from build123d import *

# Parameters (mm, degrees)
SZKIC1_W                    = 125
SZKIC1_H                    = 80
DODANIE_WYCI_GNI_CIE1_DEPTH = 12
ZAOKR_GLENIE1_R             = 5
OTW_R_POD_RUB_M81_D         = 9
OTW_R_POD_RUB_M81_DEPTH     = 16
OTW_R_POD_RUB_M81_TIP       = 2.703872786
OTW_R_POD_RUB_M82_D         = 9
OTW_R_POD_RUB_M82_DEPTH     = 16
OTW_R_POD_RUB_M82_TIP       = 2.703872786
SZKIC8_R                    = 10
WYTNIJ_WYCI_GNI_CIE1_DEPTH  = 1.5
ZAOKR_GLENIE2_R             = 1.5


with BuildPart() as part:
    # Szkic1 → Dodanie-wyciągnięcie1 (new body)
    with BuildSketch(Plane(origin=(0, 0, 0), x_dir=(1, 0, 0), z_dir=(0, 1, 0))):
        Rectangle(SZKIC1_W, SZKIC1_H)
    extrude(amount=DODANIE_WYCI_GNI_CIE1_DEPTH)

    # Zaokrąglenie1
    zaokr_glenie1_edges = [part.edges().sort_by_distance(p)[0] for p in [
        (62.5, 6, 40),
        (-62.5, 6, 40),
        (-62.5, 6, -40),
        (62.5, 6, -40),
    ]]
    fillet(zaokr_glenie1_edges, radius=ZAOKR_GLENIE1_R)

    # Otwór pod śrubę M81
    with Locations(Plane(origin=(0, 12, 0), x_dir=(1, 0, 0), z_dir=(0, 1, 0))):
        with Locations((-50, 20), (50, 20), (50, -20), (-50, -20)):
            Hole(OTW_R_POD_RUB_M81_D / 2, depth=OTW_R_POD_RUB_M81_DEPTH)
            with Locations((0, 0, -(OTW_R_POD_RUB_M81_DEPTH + OTW_R_POD_RUB_M81_TIP / 2))):  # 118° drill point
                Cone(0, OTW_R_POD_RUB_M81_D / 2, OTW_R_POD_RUB_M81_TIP, mode=Mode.SUBTRACT)

    # Otwór pod śrubę M82
    with Locations(Plane(origin=(0, 12, 0), x_dir=(1, 0, 0), z_dir=(0, 1, 0))):
        with Locations((-32.5, 32.5), (32.5, 32.5), (32.5, -32.5), (-32.5, -32.5)):
            Hole(OTW_R_POD_RUB_M82_D / 2, depth=OTW_R_POD_RUB_M82_DEPTH)
            with Locations((0, 0, -(OTW_R_POD_RUB_M82_DEPTH + OTW_R_POD_RUB_M82_TIP / 2))):  # 118° drill point
                Cone(0, OTW_R_POD_RUB_M82_D / 2, OTW_R_POD_RUB_M82_TIP, mode=Mode.SUBTRACT)

    # Szkic8 → Wytnij-wyciągnięcie1 (cut)
    with BuildSketch(Plane.XZ):
        with Locations(Location((0, 0, 0), (0, 0, 270))):
            Circle(SZKIC8_R)
    extrude(amount=-WYTNIJ_WYCI_GNI_CIE1_DEPTH, mode=Mode.SUBTRACT)

    # Zaokrąglenie2
    zaokr_glenie2_edges = [part.edges().sort_by_distance(p)[0] for p in [
        (0, 1.5, 10),
    ]]
    fillet(zaokr_glenie2_edges, radius=ZAOKR_GLENIE2_R - 0.0001)  # a hair under: the kernel refuses the full size


solid = part.part
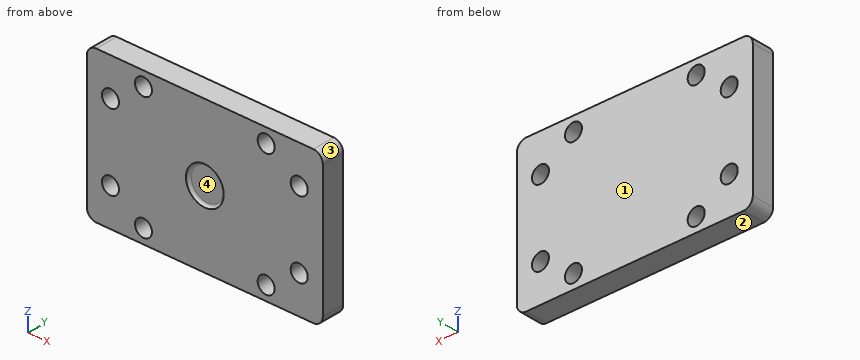
Build history of the part. All positions in model axes, mm. Face numbers are marked on the shaded views. Round coordinates to 2 decimals unless told otherwise and drop trailing zeros. Loops run counter-clockwise (first coordinate to the right, second up) from the corner with the lowest first, then second, coordinate; pieces in that order, holes last. Notation, with made-up numbers: (42.5, 78) -> (76.5, 78) arc R22 ccw to (76.5, 104) -> close; hole circle Ø5 at (60, 66). An arc over 180 degrees is marked (long way). Answer in a Markdown table with one row per item.
Item 1: Mould opens along Z. For the marked faces 1, 2, 3 and 4 say: +Z half, -Z half, draft (parallel to the pull), parting line (faces both ways), or undercut.
Answers below:
| item | result |
|---|---|
| face 1 | draft |
| face 2 | -Z half |
| face 3 | +Z half |
| face 4 | undercut |
Item 2: Drill centre lines: L1, parallel to X at y = 8.5, z = -32.5; L2, parallel to Z at x = 32.5, y = 7; L3, parallel to Z at x = -50, y = 8. Where is each one in solid material? Low to high. Write a range as [from, to].
Answers below:
| item | result |
|---|---|
| L1 | x = [-62.5, -37], [-28, 28], [37, 62.5] |
| L2 | z = [-40, -37], [-28, 28], [37, 40] |
| L3 | z = [-40, -24.5], [-15.5, 15.5], [24.5, 40] |
Item 3: Saw through at C-C (y = 8.25). State how many separate pieces and enclosed holes the cut face has, and give its area (3 significant figures).
Answers below:
| item | result |
|---|---|
| separate pieces | 1 |
| enclosed holes | 8 |
| area | 9,470 mm² |
Item 4: Saw through at B-B (x = -50). Write the cut outline in (y, z).
Answers below:
| item | result |
|---|---|
| outline | (0, -40) -> (12, -40) -> (12, -24.5) -> (0, -24.5) -> close; (0, -15.5) -> (12, -15.5) -> (12, 15.5) -> (0, 15.5) -> close; (0, 24.5) -> (12, 24.5) -> (12, 40) -> (0, 40) -> close |
Item 5: Pin check, flat tips, straight feed: pin 1 (14.5 mm diameter, centred on x = 32.5, z = 32.5, fed in from -Y); pin 2 (5 mm diameter, centred on x = 2, z = -3.5, fed in from -Y). Stop position of each tip, or through.
Answers below:
| item | result |
|---|---|
| pin 1 | stops at y = 0 |
| pin 2 | stops at y = 1.5 |
Item 6: Saw through at A-A (z = 32.5). Write the cut outline in (x, y), and give its area (3 significant figures).
Answers below:
| item | result |
|---|---|
| outline | (-62.5, 0) -> (-37, 0) -> (-37, 12) -> (-62.5, 12) -> close; (-28, 0) -> (28, 0) -> (28, 12) -> (-28, 12) -> close; (37, 0) -> (62.5, 0) -> (62.5, 12) -> (37, 12) -> close |
| area | 1,280 mm² |
